CAD build for the part. Positions are in the model's coordinates, mm. Face numbers are marked on the shaded views. A direction names the side the tool comes from. Round coordinates to 2 decimals unless told otherwise and drop trailing zeros. Order: outer loops, then holes, each group sorted by start corner. A loop starts at its lowest first (then second) coordinate and runs counter-clockwise, first axis right, second up. Notation, with made-up numbers: M 55,22.5 L 85,22.5 A28 cw 85,47.5 Z; hole C 11.5,27.25 d6. An arc over 180 degrees is marked long. Answer as a JSON object with one key per item and string values.
```python
from build123d import *

# Parameters (mm, degrees)
SZKIC1_R                         = 3.9
DODANIE_WYCI_GNI_CIE1_DEPTH      = 3
SFAZOWANIE1_SIZE                 = 2
DODANIE_WYCI_GNI_CIE2_DEPTH      = 16.75
DODANIE_WYCI_GNI_CIE2_DEPTH_BACK = 4.25


with BuildPart() as part:
    # Szkic1 → Dodanie-wyciągnięcie1 (new body)
    with BuildSketch(Plane.XY):
        Polygon((-13.75, 9.75), (-18.75, 4.75), (-18.75, -9.75), (-4.25, -9.75), (-4.25, -11.75), (16.75, -11.75), (16.75, -9.75), (18.75, -9.75), (18.75, 4.75), (13.75, 9.75), align=None)
        with Locations((8.45, 0.25)):
            Circle(SZKIC1_R, mode=Mode.SUBTRACT)
        with Locations((-10.25, 0.25)):
            Circle(SZKIC1_R, mode=Mode.SUBTRACT)
    extrude(amount=DODANIE_WYCI_GNI_CIE1_DEPTH)

    # Sfazowanie1
    sfazowanie1_edges = [part.edges().sort_by_distance(p)[0] for p in [
        (4.55, 0.25, 3),
        (-14.15, 0.25, 3),
    ]]
    chamfer(sfazowanie1_edges, length=SFAZOWANIE1_SIZE)

    # Szkic2 → Dodanie-wyciągnięcie2 (add, two sides: drawn at the far end of the back side and taken through both)
    with BuildSketch(Plane(origin=(0, 0, 0), x_dir=(0, 0, -1), z_dir=(1, 0, 0)).offset(-DODANIE_WYCI_GNI_CIE2_DEPTH_BACK)):
        with BuildLine():
            Line((-3, -11.75), (-14.433393367, -19.829450235))
            ThreePointArc((-14.433393367, -19.829450235), (-11.300096726, -30.742490463), (-7.092187095, -20.19708903))
            Line((-7.092187095, -20.19708903), (-9.705385917, -22.043715762))
            ThreePointArc((-9.705385917, -22.043715762), (-10.51292291, -27.710195248), (-13.093480354, -22.601200333))
            Line((-13.093480354, -22.601200333), (0, -13.348643413))
            Line((0, -13.348643413), (0, -11.75))
            Line((0, -11.75), (-3, -11.75))
        make_face()
    extrude(amount=DODANIE_WYCI_GNI_CIE2_DEPTH + DODANIE_WYCI_GNI_CIE2_DEPTH_BACK)


solid = part.part
```
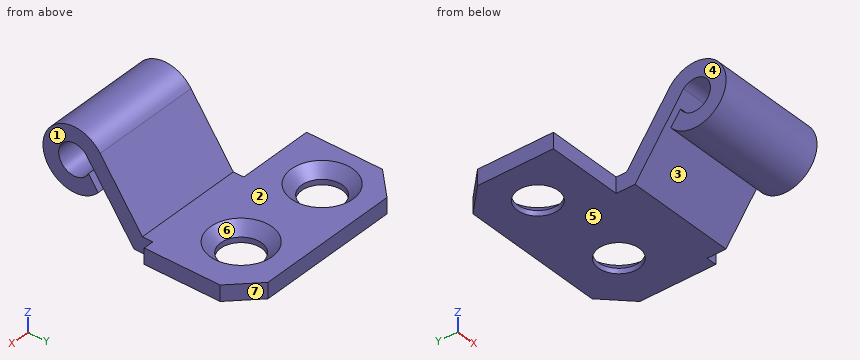
Item 1: Drop flat-ended pins along their axis: pin 1 Ø3 at (y, z) = (-26, 3) entering from -X; pin 2 Ø7 at (y, z) = (-24.75, 11) entering from +X; pin 3 Ø1 at (x, z) = (3.5, 7.5) entering from +Y; pin 4 Ø6.5 at (x, y) = (3.5, -4.5) entering from +Z. Give the stop position or say it passes through.
Worked answers:
{"pin 1": "passes through", "pin 2": "stops at x = 16.75", "pin 3": "stops at y = -14.58", "pin 4": "stops at z = 3"}
Item 2: Saw through at C-C on y = -25. List the corners of the cut face in (x, z).
Worked answers:
{"outline": "M -4.25,5.01 L 16.75,5.01 L 16.75,8.01 L -4.25,8.01 Z; M -4.25,13.99 L 16.75,13.99 L 16.75,16.99 L -4.25,16.99 Z"}
Item 3: Saw through at D-D on x = 15.5. List the corners of the cut face in (y, z), and give its area (3 significant figures).
Worked answers:
{"outline": "M -22.6,13.09 L -13.35,0 L 8,0 L 8,3 L -11.75,3 L -19.83,14.43 A6 ccw long -20.2,7.09 L -22.04,9.71 A3 cw long Z", "area": "175 mm2"}
Item 4: 3-axis set-ups, long thin cutter, end or side, ignore diameter. For the marked faces 1, 2, 3 and 4: which of +Z, -Z, +X, -X, +Y, -Y reach the whole face in a straight line?
Worked answers:
{"face 1": "+Z, -Z, +X, -Y", "face 2": "+Z, +X, -X, +Y", "face 3": "+X, -X", "face 4": "+Z, -Z, -X, -Y"}
Item 5: Saw through at B-B on z = 6. List the corners of the cut face in (x, y).
Worked answers:
{"outline": "M -4.25,-28.07 L 16.75,-28.07 L 16.75,-21.43 L -4.25,-21.43 Z; M -4.25,-17.59 L 16.75,-17.59 L 16.75,-13.87 L -4.25,-13.87 Z"}
Item 6: Saw through at A-A on x = 8.45. List the corners of the cut face in (y, z), and give its area (3 significant figures).
Worked answers:
{"outline": "M -22.6,13.09 L -13.35,0 L -3.65,0 L -3.65,1 L -5.65,3 L -11.75,3 L -19.83,14.43 A6 ccw long -20.2,7.09 L -22.04,9.71 A3 cw long Z; M 4.15,0 L 9.75,0 L 9.75,3 L 6.15,3 L 4.15,1 Z", "area": "153 mm2"}
Item 7: Two-plate mould, pull along Y, no slides. Class the marked faces 5, 6 and 7: released by +Y, released by -Y, zero draft, split by the parting line, or undercut.
Worked answers:
{"face 5": "zero draft", "face 6": "undercut", "face 7": "released by +Y"}
Item 8: Wall check: line 1 along X through (y, z) = (0.5, 1.25); line 2 along Z through (x, y) = (12.5, -25); line 3 along X through (y, z) = (-22, 9.5). Give the ranges that are in metal, low to high. Write a range as [from, to].
Worked answers:
{"line 1": "x = [-18.75, -14.39], [-6.11, 4.31], [12.59, 18.75]", "line 2": "z = [5.01, 8.01], [13.99, 16.99]", "line 3": "x = [-4.25, 16.75]"}
